Work out the finished part from the listing and answer in its coordinate system (mm). A direction names the side the tool comes from. Round coordinates to 2 decimals unless told otherwise and drop trailing zeros. Order: outer loops, then holes, each group sorted by start corner. A loop starts at its lowest first (then second) coordinate and runs counter-clockwise, first axis right, second up. Notation, with made-up numbers: (-9, -1) - (49, -1) arc R34 ccw to (49, 34) - close; hole circle Ø6 at (8, -14.5). An arc over 180 degrees is marked (long way). Use one line per item in the form item = value. Start each with the question number.
Q1. The part is cut by section C-C on z = -2. Determine the outline of the cut face in (x, y).
Q2. The part is cut by section A-A on x = 50.8. Determine the outline of the cut face in (y, z), plus the area to 3 significant figures.
Q3. Given P1, Ø6.5, axis at y = -136.5, z = 0.5, coming from the -X side; P2, Ø6.5, axis at x = -231, z = 2.5, coming from the +Y side; P3, Ø4, axis at y = 132.5, z = -1, coming from the +X side, each flat-ended and moving along its own axis, determine where each tip first touches the part or whether it passes through.
Q4. Which of the six approach directions +Z, -Z, +X, -X, +Y, -Y give full straight-line access (tool end or side, diameter ignored) to faces 1 (the flat face through (-229, -38.1, 0)), 2 (the flat face through (228, -38.1, 0)), 3 (the flat face through (-228, 38.1, 0))?
Q5. Find the intervals of material crossed by line 1 (Y direction, x = 50.8, z = 1.5); line 2 (X direction, y = -110, z = -3), in increasing order. Write a range as [from, to].
Q6. The part is cut by section D-D on y = 126. Determine the outline of the cut face in (x, z), plus the area to 3 significant figures.
Q7. The part is cut by section B-B on y = -139.7. Determine the outline of the cut face in (x, z), plus the area to 3 significant figures.
Q8. For a pull along Y with two mould halves and no side action, classify faces 4 (the flat face through (241.3, -1, 0)), 5 (the flat face through (3, 203.2, 0)), 6 (the cylindrical face through (40.7, 142.6, -0.1)), 7 (the cylindrical face through (40.7, -147.4, -0.1)) as +Y half, -Y half, draft (parallel to the pull), parting line (faces both ways), or undercut.
from build123d import *

# Parameters (mm, degrees)
BOSS_EXTRUDE1_DEPTH = 6.35
CAVITY1_START       = -6.35
CAVITY1_OUTLINE_R   = 12.7
CAVITY1_DEPTH       = 12.7


# Read off the part's stored shape, not the designer's step: Cavity1
with BuildPart() as part:
    # Sketch1 → Boss-Extrude1 (new, symmetric)
    with BuildSketch(Plane.XY):
        Polygon((-215.9, -38.1), (-215.9, -203.2), (215.9, -203.2), (215.9, -38.1), (241.3, -38.1), (241.3, 38.1), (215.9, 38.1), (215.9, 203.2), (-215.9, 203.2), (-215.9, 38.1), (-241.3, 38.1), (-241.3, -38.1), align=None)
    extrude(amount=BOSS_EXTRUDE1_DEPTH, both=True)

    # Cavity1 outline → Cavity1 (cut)
    with BuildSketch(Plane.XY.offset(CAVITY1_START)):
        with Locations((50.8, -139.7)):
            Circle(CAVITY1_OUTLINE_R)
        with Locations((50.8, 150.3)):
            Circle(CAVITY1_OUTLINE_R)
    extrude(amount=CAVITY1_DEPTH, mode=Mode.SUBTRACT)


solid = part.part
Found:
q1.outline = (-241.3, -38.1) - (-215.9, -38.1) - (-215.9, -203.2) - (215.9, -203.2) - (215.9, -38.1) - (241.3, -38.1) - (241.3, 38.1) - (215.9, 38.1) - (215.9, 203.2) - (-215.9, 203.2) - (-215.9, 38.1) - (-241.3, 38.1) - close; hole circle Ø25.4 at (50.8, -139.7); hole circle Ø25.4 at (50.8, 150.3)
q2.outline = (-203.2, -6.35) - (-152.4, -6.35) - (-152.4, 6.35) - (-203.2, 6.35) - close; (-127, -6.35) - (137.6, -6.35) - (137.6, 6.35) - (-127, 6.35) - close; (163, -6.35) - (203.2, -6.35) - (203.2, 6.35) - (163, 6.35) - close
q2.area = 4,520 mm²
q3.P1 = -215.9
q3.P2 = 38.1
q3.P3 = 215.9
q4.face_1 = +Z, -Z, -X, -Y
q4.face_2 = +Z, -Z, +X, -Y
q4.face_3 = +Z, -Z, -X, +Y
q5.line_1 = [-203.2, -152.4], [-127, 137.6], [163, 203.2]
q5.line_2 = [-215.9, 215.9]
q6.outline = (-215.9, -6.35) - (215.9, -6.35) - (215.9, 6.35) - (-215.9, 6.35) - close
q6.area = 5,480 mm²
q7.outline = (-215.9, -6.35) - (38.1, -6.35) - (38.1, 6.35) - (-215.9, 6.35) - close; (63.5, -6.35) - (215.9, -6.35) - (215.9, 6.35) - (63.5, 6.35) - close
q7.area = 5,160 mm²
q8.face_4 = draft
q8.face_5 = +Y half
q8.face_6 = undercut
q8.face_7 = undercut
